For this review, take the finished solid that the model builds, in its own axes (mm). A direction names the side the tool comes from. Give positions to 0.01 mm unless a question says otherwise; leave off trailing zeros. Loops run counter-clockwise (first coordinate to the right, second up) from the corner with the lowest first, then second, coordinate; pieces in that order, holes last. Notation, with made-up numbers: (33, 3) - (42, 3) arc R16 cw to (42, 11) - close; hole circle Ø6 at (44.25, -3). An arc over 180 degrees is marked (long way). Put each result on its own line as item: value.
from build123d import *

# Parameters (mm, degrees)
SKETCH_1_R           = 46
EXTRUDE_1_DEPTH      = 35.5
EXTRUDE_2_REACH      = 141.661
EXTRUDE_2_END_RADIUS = 46
SKETCH_2_R           = 44
SKETCH_3_W           = 10.337073316
SKETCH_3_H           = 61.617049376
SKETCH_3_W_2         = 11.195847523
CUT_EXTRUDE_1_DEPTH  = 60


with BuildPart() as part:
    # 草图1 → 凸台-拉伸1 (new, symmetric)
    with BuildSketch(Plane.XY):
        Circle(SKETCH_1_R)
    extrude(amount=EXTRUDE_1_DEPTH, both=True)

    # 凸台-拉伸2: up to this cylinder (the profile starts outside it)
    extrude_2_end = Plane(origin=(0, 0, 0), z_dir=(0, 0, -1)) * Cylinder(EXTRUDE_2_END_RADIUS, 376.322, mode=Mode.PRIVATE)
    # 草图2 → 凸台-拉伸2 (add, up to the surface)
    with BuildSketch(Plane(origin=(81, 0, 0), x_dir=(0, 0, -1), z_dir=(1, 0, 0)), mode=Mode.PRIVATE) as extrude_2_sk1:
        Circle(SKETCH_2_R)
    extrude_2_tool1 = extrude(extrude_2_sk1.sketch, amount=-EXTRUDE_2_REACH, mode=Mode.PRIVATE) - extrude_2_end
    add(extrude_2_tool1.solids().sort_by_distance((81, 0, 0))[0])

    # 草图3 → 切除-拉伸1 (cut)
    with BuildSketch(Plane(origin=(0, 0, 0), x_dir=(0, 0, -1), z_dir=(1, 0, 0))):
        with Locations((-40.668536658, 1.610201639)):
            Rectangle(SKETCH_3_W, SKETCH_3_H)
        with Locations((41.097923761, 1.610201639)):
            Rectangle(SKETCH_3_W_2, SKETCH_3_H)
    extrude(amount=CUT_EXTRUDE_1_DEPTH, mode=Mode.SUBTRACT)


solid = part.part
1) Take a section at A-A on y = 0. State the section outline as (x, z) points, and give its area (3 significant figures).
Geometry check:
outline: (-46, -35.5) - (60, -35.5) - (60, -44) - (81, -44) - (81, 44) - (60, 44) - (60, 35.5) - (-46, 35.5) - close
area: 9,370 mm²
2) For faces 1 (the face through (81, 1, 1)), 2 (the face through (60, 0, 39)), 3 (the face through (60, 0, -39)), 4 (the face through (55.19, -26.77, 34.92)), list the 3-axis set-ups (+Z, -Z, +X, -X, +Y, -Y) from which the entire face can be reached by the end or side of a thin tool; tool diameter is ignored.
Geometry check:
face 1: +Z, -Z, +X, +Y, -Y
face 2: +Z, -X, +Y, -Y
face 3: -Z, -X, +Y, -Y
face 4: +X
3) Insertion check: pin 1 Ø10 at (x, y) = (21, 35.5) entering from -Z; pin 2 Ø8 at (x, y) = (-7.5, -16.5) entering from +Z; pin 3 Ø4 at (x, z) = (32, 22.5) entering from +Y; pin 4 Ø12 at (y, z) = (-4, 7.5) entering from -X. Each pin has a flat end and moves straight along its axis. Give the tip position at first contact, or say it passes through.
Geometry check:
pin 1: stops at z = -35.5
pin 2: stops at z = 35.5
pin 3: stops at y = 38.93
pin 4: stops at x = -46
4) Take a section at D-D on x = 0. State the section outline as (y, z) points.
Geometry check:
outline: (-46, -35.5) - (46, -35.5) - (46, 35.5) - (-46, 35.5) - close
5) Take a section at B-B on x = 15.5. State the section outline as (y, z) points, and give its area (3 significant figures).
Geometry check:
outline: (-43.31, -35.5) - (43.31, -35.5) - (43.31, -7.76) arc R44 ccw to (43.31, 7.76) - (43.31, 35.5) - (-43.31, 35.5) - (-43.31, 7.76) arc R44 ccw to (-43.31, -7.76) - close
area: 6,160 mm²
6) Take a section at C-C on z = 0. State the section outline as (x, y) points.
Geometry check:
outline: (13.42, -44) - (81, -44) - (81, 44) - (13.42, 44) arc R46 ccw (long way) to start
7) Wall thickness on line 1 (Z direction, x = 8, y = -26); line 2 (Y direction, x = -1, z = -34.5); line 3 (Z direction, x = 53, y = -35.5): over which ranges is each line inside the solid? List them lowest first.
Geometry check:
line 1: z = -35.5 to 35.5
line 2: y = -45.99 to 45.99
line 3: z = -26 to 26
